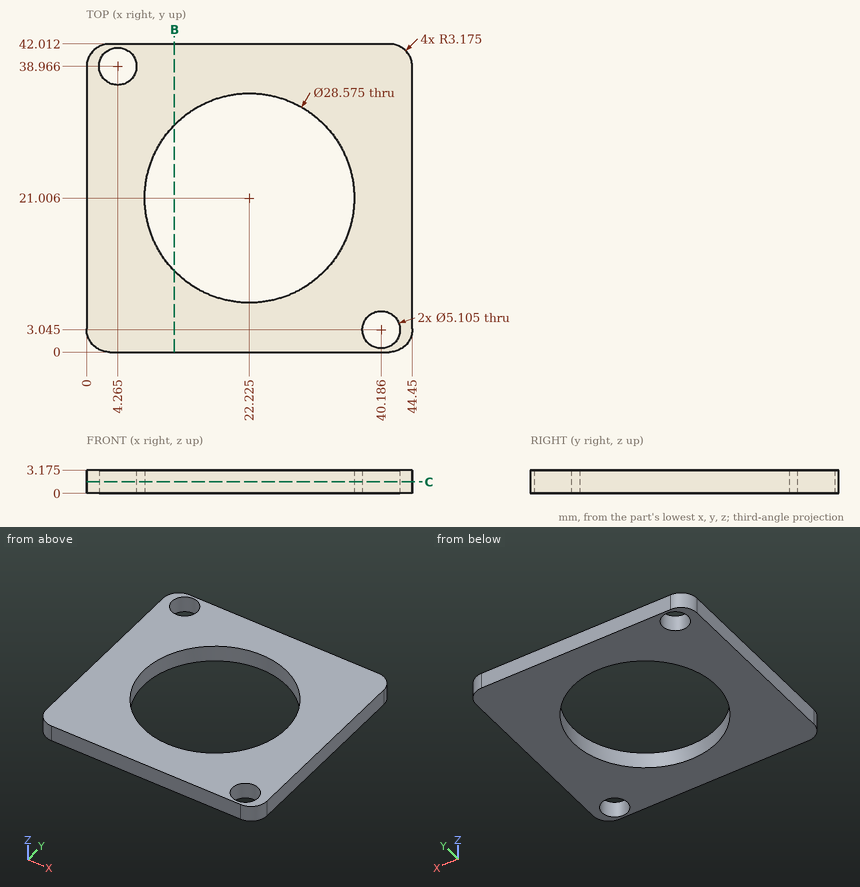
Source: three-view drawing plus pictorial views. Frame: mm from the lowest corner of the part. Give positions to 0.01 mm unless a question says otherwise; leave off trailing zeros. Write each loop counter-clockwise with the first axis right and the second up, starting at its lowest first coordinate (ties: lowest second). Pieces come first, ordered by that corner, then holes. Notation, with made-up numbers: (29.25, -22.5) - (43.25, -22.5) arc R7 cw to (43.25, -14.5) - close; hole circle Ø6 at (33, -8). An arc over 180 degrees is marked (long way). Write item = value, one per line. Start each with the question number.
Q1. Cut plane C-C, the plane z = 1.55. Give the number of separate pieces and of enclosed holes in the cut face, then the cut area to 3 significant figures.
Q2. Pin query (flat end, axial travel): pin 1 Ø4.5 at (x, y) = (40.19, 3.05) entering from -Z. Return the tip coordinate at first contact, or that it passes through.
Q3. Cut plane B-B, the plane x = 12. Return loops of the section in (y, z) (1 decimal).
Q4. Material intervals for probe 1 along Y at (x, z) = (40, 0.55); probe 2 along X at (y, z) = (40.5, 0.85) (1 decimal); probe 3 along Y at (x, z) = (35.5, 1.95) (1 decimal), sorted ascending.
Computed values:
q1.separate_pieces = 1
q1.enclosed_holes = 3
q1.area = 1,180 mm²
q2.pin_1 = through
q3.outline = (0, 0) - (11, 0) - (11, 3.2) - (0, 3.2) - close; (31, 0) - (42, 0) - (42, 3.2) - (31, 3.2) - close
q4.probe_1 = 0 to 0.5, 5.59 to 42.01
q4.probe_2 = 0.5 to 2.2, 6.3 to 44
q4.probe_3 = 0 to 15.7, 26.3 to 42
